Geometry check sheet. Reference: the model listing, model coordinates, mm. Face numbers are marked on the shaded views. Round coordinates to 2 decimals unless told otherwise and drop trailing zeros. Loops run counter-clockwise (first coordinate to the right, second up) from the corner with the lowest first, then second, coordinate; pieces in that order, holes last. Notation, with made-up numbers: M -29,29.5 L 14,29.5 A20 cw 14,63.5 Z; hole C -17,4 d11. An arc over 180 degrees is marked long. Use one line per item in the form item = value. Start each with the question number.
1. Material ranges on line 1 (X direction, y = 4.5, z = 0); line 2 (Z direction, x = -0.5, y = 5.25); line 3 (Z direction, x = -5, y = 4), recorded low to high.
2. Cross-section at B-B (x = 0). Record the boundary of the cut face in (y, z).
3. Draft check along Z on the marked faces 1, 2 and 3. Enter one of: pulls with the +Z half, pulls with the -Z half, needs draft (parallel to the pull), parting line crosses it, or undercut.
4. Cross-section at A-A (z = -2). Record the boundary of the cut face in (x, y), then the cut area to 3 significant figures.
5. Go/stop test with flat-tipped pins: pin 1 (6 mm diameter, centred on y = 8, z = 48.5, fed in from -X); pin 2 (1 mm diameter, centred on y = 5, z = 24, fed in from +X); pin 3 (1.5 mm diameter, centred on y = 7, z = 72.5, fed in from -X). Record where each tip stops, or that it passes through.
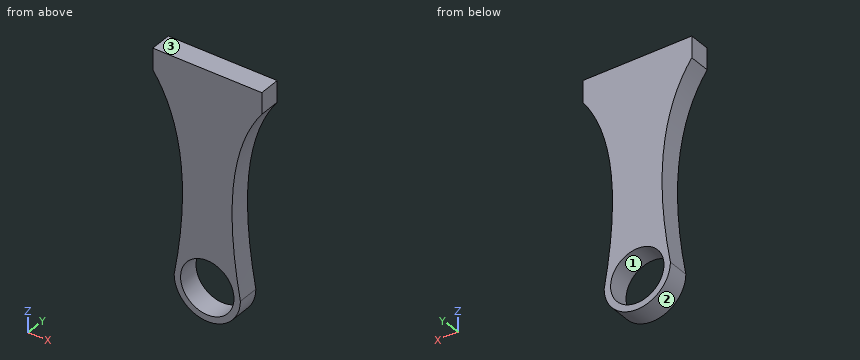
```python
from build123d import *

# Parameters (mm, degrees)
SKETCH_1_R          = 12.5
EXTRUDE_1_DEPTH     = 10
SKETCH_2_W          = 51
SKETCH_2_H          = 10
EXTRUDE_2_DEPTH     = 10
EXTRUDE_3_DEPTH     = 10
CUT_EXTRUDE_2_DEPTH = 10


with BuildPart() as part:
    # Эскиз1 → Бобышка-Вытянуть1 (new body)
    with BuildSketch(Plane(origin=(0, 0, 0), x_dir=(1, 0, 0), z_dir=(0, 1, 0))):
        with BuildLine():
            Line((-15.5, 0), (-15.5, -100))
            Line((-15.5, -100), (15.5, -100))
            Line((15.5, -100), (15.5, 0))
            ThreePointArc((15.5, 0), (0, 15.5), (-15.5, 0))
        make_face()
        with Locations(Location((0, 0, 0), (0, 0, 270))):
            Circle(SKETCH_1_R, mode=Mode.SUBTRACT)
    extrude(amount=EXTRUDE_1_DEPTH)

    # Эскиз2 → Бобышка-Вытянуть2 (add, through all)
    with BuildSketch(Plane(origin=(0, 10, 0), x_dir=(1, 0, 0), z_dir=(0, 1, 0))):
        with Locations((0, -95)):
            Rectangle(SKETCH_2_W, SKETCH_2_H)
    extrude(amount=-EXTRUDE_2_DEPTH)

    # Эскиз4 → Бобышка-Вытянуть3 (add)
    with BuildSketch(Plane(origin=(0, 10, 0), x_dir=(1, 0, 0), z_dir=(0, 1, 0))):
        Polygon((-25.5, -90), (-15.5, 0), (-15.5, -90), align=None)
        Polygon((15.5, -90), (25.5, -90), (15.5, 0), align=None)
    extrude(amount=-EXTRUDE_3_DEPTH)

    # Эскиз3 → Вырез-Вытянуть2 (cut)
    with BuildSketch(Plane(origin=(0, 10, 0), x_dir=(1, 0, 0), z_dir=(0, 1, 0))):
        with BuildLine():
            Line((-15.5, 0), (-25.5, -90))
            add(Edge.make_bspline(
                [(-15.5, 0), (-4.236810468, -61.646447202), (-25.5, -90)],
                knots=[0, 0, 0, 1, 1, 1], degree=2))
        make_face()
        with BuildLine():
            Line((15.5, 0), (25.5, -90))
            add(Edge.make_bspline(
                [(15.5, 0), (4.236810468, -61.646447202), (25.5, -90)],
                knots=[0, 0, 0, 1, 1, 1], degree=2))
        make_face()
    extrude(amount=-CUT_EXTRUDE_2_DEPTH, mode=Mode.SUBTRACT)


solid = part.part
```
Reported:
q1.line_1 = -15.5 to -12.5, 12.5 to 15.5
q1.line_2 = -15.49 to -12.49, 12.49 to 100
q1.line_3 = -14.67 to -11.46, 11.46 to 100
q2.outline = M 0,-15.5 L 10,-15.5 L 10,-12.5 L 0,-12.5 Z; M 0,12.5 L 10,12.5 L 10,100 L 0,100 Z
q3.face_1 = undercut
q3.face_2 = pulls with the -Z half
q3.face_3 = pulls with the +Z half
q4.outline = M -15.37,0 L -12.34,0 L -12.34,10 L -15.37,10 Z; M 12.34,0 L 15.37,0 L 15.37,10 L 12.34,10 Z
q4.area = 60.6 mm²
q5.pin_1 = -12.18
q5.pin_2 = 12.28
q5.pin_3 = -16.73
